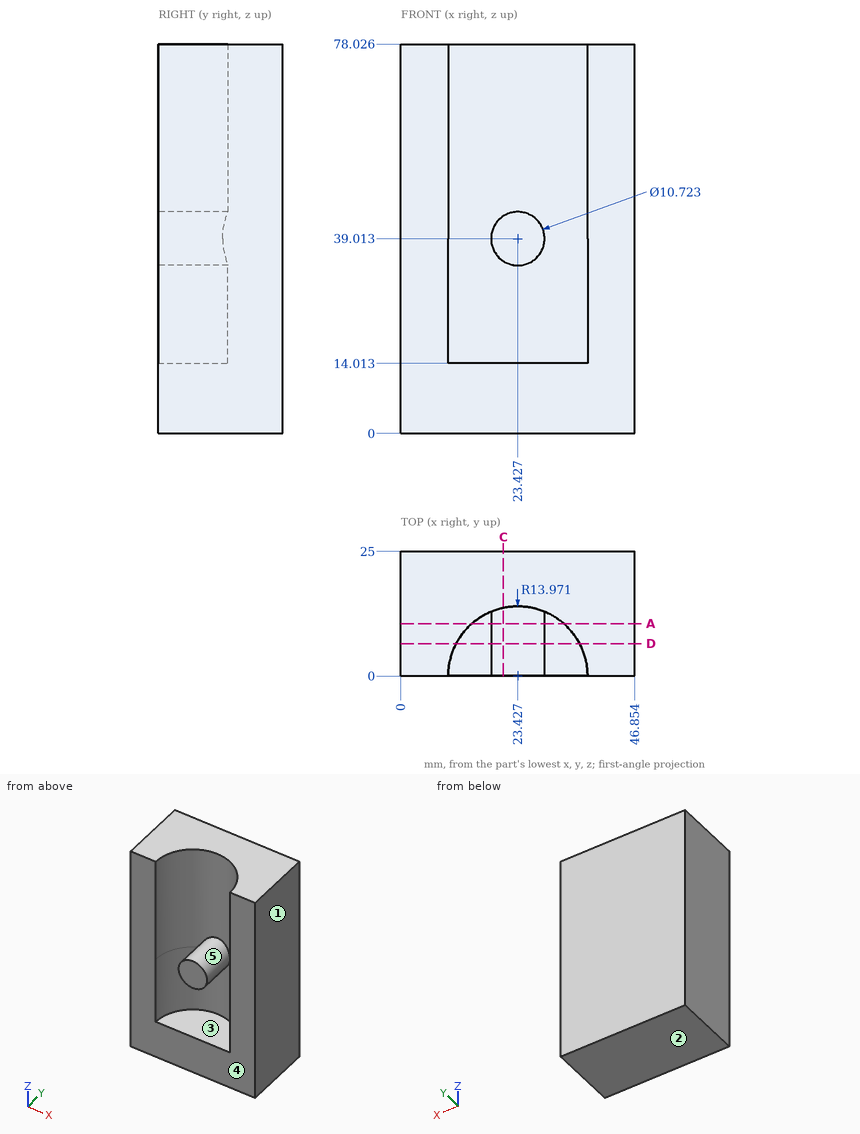
Check sheet for the drawn part. Datum: minimum x, y, z corner. Units: mm. A direction names the side the tool comes from. Round coordinates to 2 decimals unless told otherwise and drop trailing zeros. Order: outer loops, then holes, each group sorted by start corner. A loop starts at its lowest first (then second) coordinate and runs counter-clockwise, first axis right, second up.
1) Tool access check on the marked faces 4 and 5. Record the directions out of +Z, -Z, +X, -X, +Y, -Y that give a thin tool (end or side, any length) a straight path to the whole face; none if there is none.
2) Section check A-A (y = 10.5). Record the boundary of the cut face in (x, z).
3) Go/stop test with flat-tipped pins: pin 1 Ø1 at (x, y) = (12.5, 15.5) entering from -Z; pin 2 Ø4 at (x, y) = (29, 7) entering from +Z. Record where each tip stops, or that it passes through.
4) Mould release check, pull along X, two halves, no side actions. Record for the marked faces 1, 2 and 3: +X half, -X half, draft (parallel to the pull), parting line (faces both ways), or undercut.
5) Section check C-C (x = 20.5). Record the boundary of the cut face in (y, z) (1 decimal).
6) Section check D-D (y = 6.5). Record the boundary of the cut face in (x, z).
7) Scan lines: line 1 (X direction, y = 9, z = 40.5) (1 decimal); line 2 (X direction, y = 9, z = 40) (1 decimal); line 3 (X direction, y = 9, z = 60) (1 decimal). Record each from-to range of solid material in increasing order.
Result:
1. face 4: +Z, -Z, +X, -X, -Y
1. face 5: -Y
2. outline: (0, 0) - (46.85, 0) - (46.85, 78.03) - (32.64, 78.03) - (32.64, 14.01) - (14.21, 14.01) - (14.21, 78.03) - (0, 78.03) - close; circle Ø10.72 at (23.43, 39.01)
3. pin 1: stops at z = 0
3. pin 2: stops at z = 43.01
4. face 1: +X half
4. face 2: draft
4. face 3: undercut
5. outline: (0, 0) - (25, 0) - (25, 78) - (13.7, 78) - (13.7, 43.5) - (0, 43.5) - (0, 34.5) - (13.7, 34.5) - (13.7, 14) - (0, 14) - close
6. outline: (0, 0) - (46.85, 0) - (46.85, 78.03) - (35.79, 78.03) - (35.79, 14.01) - (11.06, 14.01) - (11.06, 78.03) - (0, 78.03) - close; circle Ø10.72 at (23.43, 39.01)
7. line 1: x = 0 to 12.7, 18.3 to 28.6, 34.1 to 46.9
7. line 2: x = 0 to 12.7, 18.2 to 28.7, 34.1 to 46.9
7. line 3: x = 0 to 12.7, 34.1 to 46.9
